Drawing for the job (mm, zero at the part's lowest x, y, z). A direction names the side the tool comes from. Give positions to 0.01 mm unless a question says otherwise; leave off trailing zeros. Loops run counter-clockwise (first coordinate to the right, second up) from the corner with the lowest first, then second, coordinate; pieces in that order, holes last. Notation, with made-up numbers: (11, -21.5) -> (39, -21.5) arc R18 cw to (39, -8.5) -> close; hole circle Ø9 at (39, 73.25). An arc over 180 degrees is marked (long way). Use CSV: the item, a comma, the result in double quotes. Start each with the question number.
(1) 3-axis set-ups, long thin cutter, end or side, ignore diameter. For the marked faces 1 and 2: which of +Z, -Z, +X, -X, +Y, -Y reach the whole face in a straight line?
(2) Cut at D-D on x = 24.5. Write the cut outline in (y, z), then the cut area to 3 significant figures.
(3) Flat gauge pins, fed straight in: pin 1 (4 mm diameter, centred on x = 21.5, z = 19, fed in from +Y); pin 2 (5 mm diameter, centred on x = 6.35, z = 19.05, fed in from +Y); pin 3 (7.5 mm diameter, centred on x = 31.5, y = 21, fed in from +Z); pin 4 (1 mm diameter, centred on x = 37.5, y = 15.5, fed in from -Z). Where does each tip first touch, or does it go through?
(4) Cut at B-B on z = 19.05. Write the cut outline in (x, y), then the cut area to 3 significant figures.
(5) Drill centre lines: probe 1 along X at (y, z) = (4.25, 19.05); probe 2 along Z at (x, y) = (6.35, 6); probe 3 along Y at (x, z) = (12.7, 2.5). Where is each one in solid material? Low to high.
(6) Cut at C-C on y = 19.05. Write the cut outline in (x, z), then the cut area to 3 significant figures.
(7) Cut at A-A on x = 38.1. Write the cut outline in (y, z).
(8) Pull direction Y, two halves, no side cores. Call the marked faces 3, 4 and 5: pulls with the +Y half, pulls with the -Y half, needs draft (parallel to the pull), parting line crosses it, or undercut.
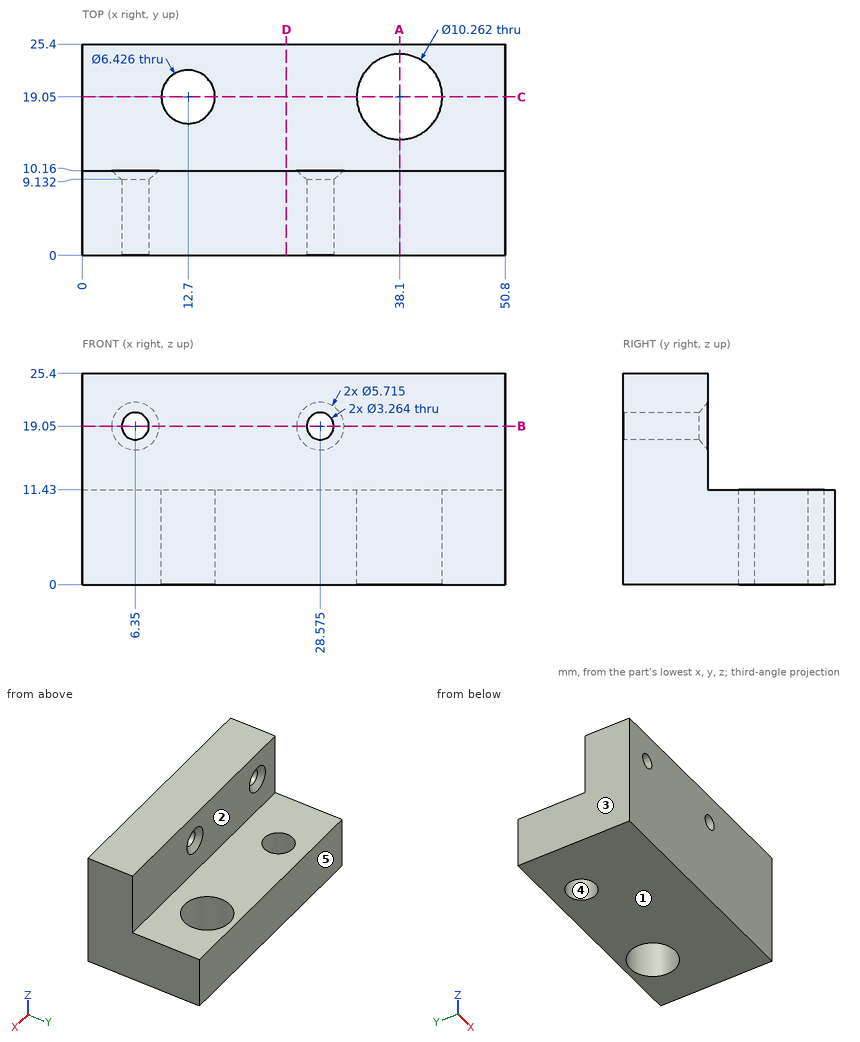
Check result:
1,face 1,"-Z, +X, -X, +Y, -Y"
1,face 2,"+Z, +X, -X, +Y"
2,outline,"(0, 0) -> (25.4, 0) -> (25.4, 11.43) -> (10.16, 11.43) -> (10.16, 25.4) -> (0, 25.4) -> close"
2,area,"432 mm²"
3,pin 1,"y = 10.16"
3,pin 2,"y = 9.86"
3,pin 3,"z = 11.43"
3,pin 4,"through"
4,outline,"(0, 0) -> (4.72, 0) -> (4.72, 9.13) -> (3.49, 10.16) -> (0, 10.16) -> close; (7.98, 0) -> (26.94, 0) -> (26.94, 9.13) -> (25.72, 10.16) -> (9.21, 10.16) -> (7.98, 9.13) -> close; (30.21, 0) -> (50.8, 0) -> (50.8, 10.16) -> (31.43, 10.16) -> (30.21, 9.13) -> close"
4,area,"447 mm²"
5,probe 1,"0 to 4.72, 7.98 to 26.94, 30.21 to 50.8"
5,probe 2,"0 to 17.42, 20.68 to 25.4"
5,probe 3,"0 to 15.84, 22.26 to 25.4"
6,outline,"(0, 0) -> (9.49, 0) -> (9.49, 11.43) -> (0, 11.43) -> close; (15.91, 0) -> (32.97, 0) -> (32.97, 11.43) -> (15.91, 11.43) -> close; (43.23, 0) -> (50.8, 0) -> (50.8, 11.43) -> (43.23, 11.43) -> close"
6,area,"390 mm²"
7,outline,"(0, 0) -> (13.92, 0) -> (13.92, 11.43) -> (10.16, 11.43) -> (10.16, 25.4) -> (0, 25.4) -> close; (24.18, 0) -> (25.4, 0) -> (25.4, 11.43) -> (24.18, 11.43) -> close"
8,face 3,"needs draft"
8,face 4,"undercut"
8,face 5,"pulls with the +Y half"
